Model file for the job. Use its own axes, mm. Face numbers are marked on the shaded views. Coordinates: 2 decimals unless noted, no trailing zeros. Write each loop counter-clockwise with the first axis right and the second up, starting at its lowest first coordinate (ties: lowest second). Pieces come first, ordered by that corner, then holes. Notation, with made-up numbers: (-21.75, 64) - (8.25, 64) arc R14 ccw to (8.25, 86) - close; hole circle Ø10 at (-24, -3.75). An arc over 180 degrees is marked (long way). Put each result on its own line as item: value. Start each with the question number.
1. Drill centre lines: L1, parallel to X at y = -122.5, z = -231; L2, parallel to X at y = 518, z = -299; L3, parallel to Z at x = 134, y = 345. Where is each one in solid material? Low to high. Write a range as from..to.
2. Saw through at A-A, the plane y = -199. Write the cut outline in (x, z), plus the area to 3 significant figures.
3. Pull direction X, two halves, no side cores. Call the marked faces 1, 2 and 3: released by +X, released by -X, zero draft, split by the parting line, or undercut.
4. Drop flat-ended pins along their axis: P1, Ø2, axis at y = -31, z = -472, coming from the -X side; P2, Ø2, axis at x = -693.5, y = 261.5, coming from the +Z side; P3, Ø2, axis at y = -115, z = -202, coming from the -X side. Give the stop position or say it passes through.
5. Saw through at C-C, the plane x = 231. Write the cut outline in (y, z), plus the area to 3 significant figures.
6. Saw through at D-D, the plane z = -341. Write the cut outline in (x, y), plus the area to 3 significant figures.
7. Saw through at B-B, the plane z = -167. Write the cut outline in (x, y), plus the area to 3 significant figures.
```python
from build123d import *

# Parameters (mm, degrees)
BOSS_EXTRUDE1_DEPTH = 6.35
BOSS_EXTRUDE2_DEPTH = 6.35
CUT_EXTRUDE2_REACH  = 932.677
BOSS_EXTRUDE3_DEPTH = 889


with BuildPart() as part:
    # Sketch3 → Boss-Extrude1 (new body)
    with BuildSketch(Plane(origin=(0, 0, 0), x_dir=(0, 0, -1), z_dir=(1, 0, 0))):
        Polygon((0, 0), (635, 0), (635, 609.6), (0, 501.65), align=None)
    extrude(amount=BOSS_EXTRUDE1_DEPTH)

    # Sketch5 → Boss-Extrude2 (add)
    with BuildSketch(Plane(origin=(0, 487.559529595, 82.885120031), x_dir=(1, 0, 0), z_dir=(0, 0.985855847, 0.167595494))):
        Polygon((6.35, 84.074279532), (378.227310637, 728.184675737), (-924.327310637, 728.184675737), (-552.45, 84.074279532), align=None)
    extrude(amount=BOSS_EXTRUDE2_DEPTH)

    # Sketch10 → Cut-Extrude2 (cut, up to next)
    with BuildSketch(Plane(origin=(6.35, 0, 0), x_dir=(0, 0, -1), z_dir=(1, 0, 0)), mode=Mode.PRIVATE) as cut_extrude2_sk1:
        Polygon((0, 501.65), (0, 0), (635, 0), (635, 609.6), align=None)
    cut_extrude2_tool1 = extrude(cut_extrude2_sk1.sketch, amount=-CUT_EXTRUDE2_REACH, mode=Mode.PRIVATE) & part.part
    add(cut_extrude2_tool1.solids().sort_by_distance((6.35, 278.686381, -327.780952))[0], mode=Mode.SUBTRACT)

    # Sketch9 → Boss-Extrude3 (add)
    with BuildSketch(Plane(origin=(0, 487.559529595, 82.885120031), x_dir=(1, 0, 0), z_dir=(0, -0.985855847, -0.167595494))):
        Polygon((378.227310637, -728.184675737), (6.35, -84.074279532), (-0.982348419, -84.074279532), (370.894962218, -728.184675737), align=None)
        Polygon((-924.327310637, -728.184675737), (-552.45, -84.074279532), (-545.117651581, -84.074279532), (-916.994962218, -728.184675737), align=None)
    extrude(amount=BOSS_EXTRUDE3_DEPTH)


solid = part.part
```
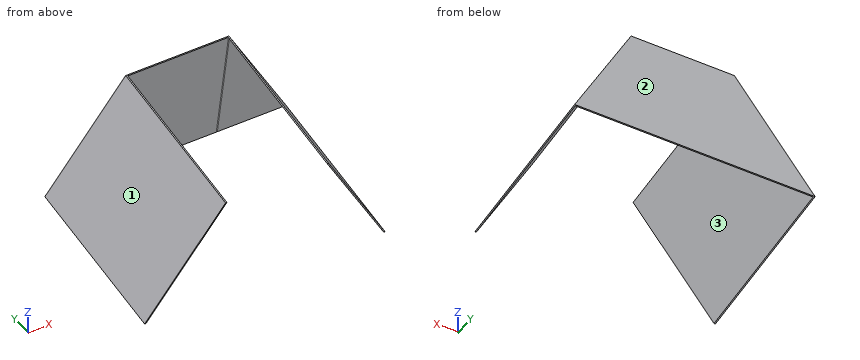
Final values:
1. L1: x = -623.54..-616.21, 70.11..77.44
1. L2: x = -724.22..-716.89, 170.79..178.12
1. L3: z = -263.78..-250.9
2. outline: (-924.33, -772.46) - (-916.99, -772.46) - (-545.12, -119.11) - (-552.45, -119.11) - close; (-0.98, -119.11) - (370.89, -772.46) - (378.23, -772.46) - (6.35, -119.11) - close
2. area: 9,580 mm²
3. face 1: released by -X
3. face 2: zero draft
3. face 3: undercut
4. P1: stops at x = -770.14
4. P2: stops at z = -286.87
4. P3: stops at x = -608.33
5. outline: (-309.56, -532.59) - (-307.44, -545.11) - (568.99, -396.12) - (609.6, -635) - (615.86, -633.94) - (573.12, -382.54) - close
5. area: 12,900 mm²
6. outline: (-752.77, 566.06) - (-664.9, -342.13) - (-657.56, -342.13) - (-744.82, 559.62) - (198.72, 559.62) - (111.46, -342.13) - (118.8, -342.13) - (206.67, 566.06) - close
6. area: 19,400 mm²
7. outline: (-650.87, 536.48) - (-563, -371.71) - (-555.66, -371.71) - (-642.92, 530.04) - (96.82, 530.04) - (9.56, -371.71) - (16.9, -371.71) - (104.77, 536.48) - close
7. area: 18,100 mm²
